For this review, take the finished solid that the model builds, in its own axes (mm). Face numbers are marked on the shaded views. A direction names the side the tool comes from. Round coordinates to 2 decimals unless told otherwise and drop trailing zeros. Write each loop counter-clockwise with the first axis right and the second up, starting at its lowest first coordinate (ties: lowest second). Pieces come first, ordered by that corner, then holes. Notation, with made-up numbers: (44, 80.5) -> (57, 80.5) arc R12 cw to (57, 94.5) -> close; hole circle Ø1 at (20, -9.75). An arc over 180 degrees is marked (long way). Answer as CSV lines item,"result". Start each with the question number.
Item 1: Mouldability with a two-part tool opening along Y and no side actions: class the marked faces 5, 6, 7 and 8 as +Y half, -Y half, draft (parallel to the pull), parting line (faces both ways), or undercut.
Item 2: Take a section at A-A on y = -33. Give the boundary of the cut face in (x, z).
Item 3: Take a section at D-D on y = -7. Give the boundary of the cut face in (x, z), then the cut area to 3 significant figures.
Item 4: For pin 1 Ø1.8 at (y, z) = (2.5, 3) entering from +X; pin 2 Ø1 at (x, z) = (38, 1.5) entering from +Y; pin 3 Ø3 at (x, z) = (-5.5, 4) entering from -Y, all flat-tipped, find the tip position at first contact; note any pin that passes through.
Item 5: Wall thickness on probe 1 along Y at (x, z) = (25, 2.85); probe 2 along X at (y, z) = (-41, 2.9); probe 3 along X at (y, z) = (-46, 1.6): over which ranges is each line inside the solid? List them lowest first. Write a range as from..to.
Item 6: Take a section at C-C on y = -14.5. Give the boundary of the cut face in (x, z).
Item 7: Take a section at B-B on x = -6. Give the boundary of the cut face in (y, z).
Item 8: Machinability: for the marked faces 1, 2, 3 and 4, which of the approach directions +Z, -Z, +X, -X, +Y, -Y give a long, thin tool a straight path to every point of the face, cutting with its end or side? Answer none if there is none.
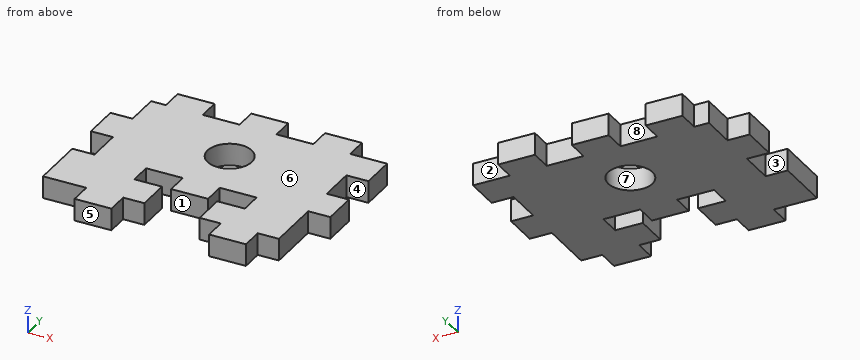
Autodesk Inventor part; units mm, degrees
ref_plane "YZ Plane" through (0, 0, 0) normal (1, 0, 0) x (0, 1, 0)
ref_plane "XZ Plane" through (0, 0, 0) normal (0, 1, 0) x (-1, 0, 0)
ref_plane "XY Plane" through (0, 0, 0) normal (0, 0, 1) x (1, 0, 0)
ref_plane "Work Plane1" through (20, 0, 0) normal (0, 0, 1) x (1, 0, 0)
sketch "Sketch1" plane through (20, 0, 0) normal (0, 0, 1) x (1, 0, 0)
  line L0 (-20, 0) -> (-10, 0)
  line L1 (-10, 0) -> (-10, 6)
  line L2 (-20, 6) -> (-10, 6)
  line L3 (-20, 0) -> (-20, 6)
  line L4 (0, 0) -> (10, 0)
  line L5 (10, 0) -> (10, 6)
  line L6 (0, 6) -> (10, 6)
  line L7 (0, 0) -> (0, 6)
  line L8 (20, 0) -> (30, 0)
  line L9 (30, 0) -> (30, 6)
  line L10 (20, 6) -> (30, 6)
  line L11 (20, 0) -> (20, 6)
  line L12 (-30, 0) -> (-24, 0)
  line L13 (-24, 0) -> (-24, 6)
  line L14 (-30, 6) -> (-24, 6)
  line L15 (-30, 0) -> (-30, 6)
  line L16 (-30, 0) -> (-20, 0)
  line L17 (-10, 0) -> (0, 0)
  line L18 (10, 0) -> (20, 0)
  line L19 (30, 0) -> (40, 0)
  line L20 (40, 0) -> (-24, 0)
  line L21 (-24, 0) -> (-24, -29)
  line L22 (-24, -29) -> (40, -29)
  line L23 (40, -29) -> (40, 0)
  line L24 (-24, -9.5) -> (-30, -9.5)
  line L25 (-30, -9.5) -> (-30, -19.5)
  line L26 (-30, -19.5) -> (-24, -19.5)
  line L27 (-24, -19.5) -> (-24, -9.5)
  line L28 (40, -19.5) -> (34, -19.5)
  line L29 (34, -19.5) -> (34, -9.5)
  line L30 (34, -9.5) -> (40, -9.5)
  line L31 (40, -9.5) -> (40, -19.5)
  line L32 (-24, -14.5) -> (40, -14.5) construction
  line L33 (-20, -29) -> (-10, -29)
  line L34 (-10, -29) -> (-10, -35)
  line L35 (-20, -35) -> (-10, -35)
  line L36 (-20, -29) -> (-20, -35)
  line L37 (0, -29) -> (10, -29)
  line L38 (10, -29) -> (10, -35)
  line L39 (0, -35) -> (10, -35)
  line L40 (0, -29) -> (0, -35)
  line L41 (20, -29) -> (30, -29)
  line L42 (30, -29) -> (30, -35)
  line L43 (20, -35) -> (30, -35)
  line L44 (20, -29) -> (20, -35)
  line L45 (-10, -29) -> (0, -29)
  line L46 (10, -29) -> (20, -29)
  point P0 (-30, -14.5)
  point P1 (34, -14.5)
  dimension "d0" = 29
  dimension "d1" = 6
  dimension "d2" = 10
extrude "Plate1" add sketch "Sketch1" along normal blind 6 contours L3 L2 L1 L0 | L0 L17 L4 L18 L8 L19 L23 L30 L29 L28 L22 L21 L16 | L7 L6 L5 L4 | L21 L26 L25 L24 | L11 L10 L9 L8 | L22 L34 L35 L36 | L22 L38 L39 L40 | L22 L42 L43 L44
sketch "Sketch2" plane through (20, 0, 6) normal (0, 0, 1) x (1, 0, 0)
  line L0 (-24, -44) -> (-24, -29)
  line L1 (-18.25, -44) -> (-30, -44)
  line L2 (-2.5, -44) -> (-8.25, -44)
  line L3 (-2.5, -35.5) -> (-2.5, -44)
  line L4 (12, -35) -> (-2, -35)
  line L5 (10, -35) -> (0, -35) construction
  line L6 (5, -35) -> (5, 6) construction
  line L7 (0, 6) -> (10, 6) construction
  line L8 (40, -19.5) -> (34, -19.5)
  line L9 (34, -19.5) -> (34, -9.5)
  line L10 (34, -9.5) -> (40, -9.5)
  line L11 (40, 0) -> (40, -9.5)
  line L12 (30, 0) -> (40, 0)
  line L13 (30, 6) -> (30, 0)
  line L14 (20, 6) -> (30, 6)
  line L15 (20, 0) -> (20, 6)
  line L16 (10, 0) -> (20, 0)
  line L17 (10, 6) -> (10, 0)
  line L18 (0, 6) -> (10, 6)
  line L19 (0, 0) -> (0, 6)
  line L20 (-10, 0) -> (0, 0)
  line L21 (-10, 6) -> (-10, 0)
  line L22 (-20, 6) -> (-10, 6)
  line L23 (-20, 0) -> (-20, 6)
  line L24 (-24, 0) -> (-20, 0)
  line L25 (-24, -9.5) -> (-24, 0)
  line L26 (-30, -9.5) -> (-24, -9.5)
  line L27 (-30, -19.5) -> (-30, -9.5)
  line L28 (-24, -19.5) -> (-30, -19.5)
  line L29 (-24, -29) -> (-24, -19.5)
  line L30 (-20, -29) -> (-24, -29)
  line L31 (-20, -35) -> (-20, -29)
  line L32 (-10, -35) -> (-20, -35)
  line L33 (-10, -29) -> (-10, -35)
  line L34 (0, -29) -> (-10, -29)
  line L35 (0, -35) -> (0, -29)
  line L36 (10, -35) -> (0, -35)
  line L37 (10, -29) -> (10, -35)
  line L38 (20, -29) -> (10, -29)
  line L39 (20, -35) -> (20, -29)
  line L40 (30, -35) -> (20, -35)
  line L41 (30, -29) -> (30, -35)
  line L42 (40, -29) -> (30, -29)
  line L43 (40, -19.5) -> (40, -29)
  line L44 (-2.5, -44) -> (-2.5, -35)
  line L45 (-2.5, -35) -> (0, -35)
  line L46 (-8.25, -50) -> (-18.25, -50)
  line L47 (-18.25, -50) -> (-18.25, -44)
  line L48 (34, -44) -> (34, -29)
  line L49 (12.5, -44) -> (18.25, -44)
  line L50 (12.5, -35.5) -> (12.5, -44)
  line L51 (30, -29) -> (34, -29)
  line L52 (30, -35) -> (30, -29)
  line L53 (20, -35) -> (30, -35)
  line L54 (20, -29) -> (20, -35)
  line L55 (10, -29) -> (20, -29)
  line L56 (10, -35) -> (10, -29)
  line L57 (12.5, -44) -> (12.5, -35)
  line L58 (12.5, -35) -> (10, -35)
  line L59 (18.25, -50) -> (28.25, -50)
  line L60 (28.25, -50) -> (28.25, -44)
  line L61 (28.25, -44) -> (34, -44)
  line L62 (-24, -29) -> (-20, -29)
  line L63 (-20, -35) -> (-20, -29)
  line L64 (-20, -35) -> (-20, -29)
  line L65 (-20, -35) -> (-10, -35)
  line L66 (-10, -35) -> (-10, -29)
  line L67 (0, -29) -> (-10, -29)
  line L68 (0, -29) -> (0, -35)
  line L69 (-8.25, -44) -> (-8.25, -50)
  line L70 (18.25, -50) -> (18.25, -44)
  line L71 (34, -44) -> (34, -29)
  line L72 (28.25, -44) -> (40, -44)
  line L73 (12.5, -44) -> (18.25, -44)
  line L74 (12.5, -35.5) -> (12.5, -44)
  line L75 (30, -29) -> (34, -29)
  line L76 (30, -35) -> (30, -29)
  line L77 (20, -35) -> (30, -35)
  line L78 (20, -29) -> (20, -35)
  line L79 (10, -29) -> (20, -29)
  line L80 (10, -35) -> (10, -29)
  line L81 (12.5, -44) -> (12.5, -35)
  line L82 (12.5, -35) -> (10, -35)
  line L83 (18.25, -50) -> (28.25, -50)
  line L84 (28.25, -50) -> (28.25, -44)
  line L85 (34, -29) -> (30, -29)
  line L86 (30, -35) -> (30, -29)
  line L87 (30, -35) -> (30, -29)
  line L88 (30, -35) -> (20, -35)
  line L89 (20, -35) -> (20, -29)
  line L90 (10, -29) -> (20, -29)
  line L91 (10, -29) -> (10, -35)
  line L92 (18.25, -44) -> (18.25, -50)
  line L93 (-24, -44) -> (-30, -44)
  line L94 (-30, -44) -> (-30, -29)
  line L95 (-30, -29) -> (-24, -29)
  line L96 (-24, -29) -> (-24, -44)
  line L97 (-10, -29) -> (0, -29)
  line L98 (0, -29) -> (0, -35)
  line L99 (0, -35) -> (-10, -35)
  line L100 (-10, -35) -> (-10, -29)
  line L101 (20, -29) -> (10, -29)
  line L102 (10, -29) -> (20, -29)
  line L103 (20, -29) -> (20, -35)
  line L104 (20, -35) -> (10, -35)
  line L105 (10, -35) -> (10, -29)
  line L106 (30, -29) -> (34, -29)
  line L107 (34, -29) -> (34, -35)
  line L108 (34, -35) -> (30, -35)
  line L109 (30, -35) -> (30, -29)
  line L110 (-20, -29) -> (-24, -29)
  line L111 (-24, -29) -> (-24, -35)
  line L112 (-24, -35) -> (-20, -35)
  line L113 (-20, -35) -> (-20, -29)
  line L114 (30, -35) -> (20, -35)
  point P0 (-2.5, -49.5)
  point P1 (12.5, -49.5)
  point P2 (12.5, -49.5)
  dimension "d4" = 10
  dimension "d6" = 6
  dimension "d12" = 6
  dimension "d13" = 15
sheet face with bend "Face2" sketch "Sketch2" thickness 6 toward (0, 0, -1) bend radius 6 contours L1 L94 L95 L0 | L0 L112 L32 L99 L44 L3 L2 L69 L46 L47 L1 | L0 L30 L31 L112 | L104 L40 L108 L48 L61 L60 L59 L70 L49 L50 L57 | L41 L42 L48 L108
bend "Bend1"
sketch "Sketch3" plane through (20, 0, 6) normal (0, 0, 1) x (1, 0, 0)
  line L0 (40, -19.5) -> (34, -19.5)
  line L1 (34, -19.5) -> (34, -9.5)
  line L2 (34, -9.5) -> (40, -9.5)
  line L3 (40, 0) -> (40, -9.5)
  line L4 (30, 0) -> (40, 0)
  line L5 (30, 6) -> (30, 0)
  line L6 (20, 6) -> (30, 6)
  line L7 (20, 0) -> (20, 6)
  line L8 (10, 0) -> (20, 0)
  line L9 (10, 6) -> (10, 0)
  line L10 (0, 6) -> (10, 6)
  line L11 (0, 0) -> (0, 6)
  line L12 (-10, 0) -> (0, 0)
  line L13 (-10, 6) -> (-10, 0)
  line L14 (-20, 6) -> (-10, 6)
  line L15 (-20, 0) -> (-20, 6)
  line L16 (-24, 0) -> (-20, 0)
  line L17 (-24, -9.5) -> (-24, 0)
  line L18 (-30, -9.5) -> (-24, -9.5)
  line L19 (-30, -19.5) -> (-30, -9.5)
  line L20 (-24, -19.5) -> (-30, -19.5)
  line L21 (-24, -29) -> (-24, -19.5)
  line L22 (-24, -29) -> (-30, -29)
  line L23 (-30, -29) -> (-30, -44)
  line L24 (-30, -44) -> (-18.25, -44)
  line L25 (-18.25, -44) -> (-18.25, -50)
  line L26 (-18.25, -50) -> (-8.25, -50)
  line L27 (-8.25, -50) -> (-8.25, -44)
  line L28 (-8.25, -44) -> (-2.5, -44)
  line L29 (-2.5, -44) -> (-2.5, -35)
  line L30 (-2.5, -35) -> (-10, -35)
  line L31 (-10, -29) -> (-10, -35)
  line L32 (0, -29) -> (-10, -29)
  line L33 (0, -35) -> (0, -29)
  line L34 (10, -35) -> (0, -35)
  line L35 (10, -29) -> (10, -35)
  line L36 (20, -29) -> (10, -29)
  line L37 (20, -35) -> (20, -29)
  line L38 (20, -35) -> (12.5, -35)
  line L39 (12.5, -35) -> (12.5, -44)
  line L40 (12.5, -44) -> (18.25, -44)
  line L41 (18.25, -44) -> (18.25, -50)
  line L42 (18.25, -50) -> (28.25, -50)
  line L43 (28.25, -50) -> (28.25, -44)
  line L44 (28.25, -44) -> (34, -44)
  line L45 (34, -44) -> (34, -29)
  line L46 (40, -29) -> (34, -29)
  line L47 (40, -19.5) -> (40, -29)
  circle A0 centre (5, -14.5) radius 6
  point P0 (5, 6)
  point P1 (34, -14.5)
  dimension "d14" = 12
extrude "Cut1" cut sketch "Sketch3" against normal blind 6 contours A0
equation "\"d12\" = d6"
equation "\"d15\" = Thickness"
equation "\"d3\" = Thickness"
equation "\"d7\" = BendRadius"
equation "\"d8\" = BendReliefWidth"
equation "\"d10\" = MinimumRemnant"
equation "\"d9\" = BendReliefDepth"
equation "\"d11\" = TransitionRadius"
equation "\"BendRadius\" = Thickness"
equation "\"BendReliefWidth\" = Thickness"
equation "\"BendReliefDepth\" = 0.5 * Thickness"
equation "\"CornerReliefSize\" = 4 * Thickness"
equation "\"MinimumRemnant\" = 2 * Thickness"
equation "\"TransitionRadius\" = BendRadius"
equation "\"JacobiRadiusSize\" = BendRadius"
equation "\"GapSize\" = Thickness"
properties part number "jotstick behuizing zijkant 2.1" material "Wood (Birch)"
Output values:
1,face 5,"-Y half"
1,face 6,"draft"
1,face 7,"undercut"
1,face 8,"+Y half"
2,outline,"(-10, 0) -> (10, 0) -> (10, 6) -> (-10, 6) -> close; (20, 0) -> (30, 0) -> (30, 6) -> (20, 6) -> close; (40, 0) -> (54, 0) -> (54, 6) -> (40, 6) -> close"
3,outline,"(-4, 0) -> (60, 0) -> (60, 6) -> (-4, 6) -> close"
3,area,"384 mm^2"
4,pin 1,"stops at x = 50"
4,pin 2,"stops at y = 0"
4,pin 3,"stops at y = -44"
5,probe 1,"y = -35..-20.5, -8.5..6"
5,probe 2,"x = -10..17.5, 32.5..54"
5,probe 3,"x = 1.75..11.75, 38.25..48.25"
6,outline,"(-10, 0) -> (19, 0) -> (19, 6) -> (-10, 6) -> close; (31, 0) -> (54, 0) -> (54, 6) -> (31, 6) -> close"
7,outline,"(-44, 0) -> (-29, 0) -> (-29, 6) -> (-44, 6) -> close; (-19.5, 0) -> (-9.5, 0) -> (-9.5, 6) -> (-19.5, 6) -> close"
8,face 1,"+Z, -Z, -Y"
8,face 2,"+Z, -Z, +X, +Y"
8,face 3,"+Z, -Z, -X"
8,face 4,"+Z, -Z, +X"
